```python
from build123d import *

# Parameters (mm, degrees)
BOSS_EXTRUDE1_DEPTH = 200
SKETCH2_R           = 2.5
CUT_EXTRUDE2_DEPTH  = 15
CUT_EXTRUDE3_START  = -15
SKETCH3_R           = 2.5
CUT_EXTRUDE3_DEPTH  = 15


with BuildPart() as part:
    # Sketch1 → Boss-Extrude1 (new body)
    with BuildSketch(Plane.XY):
        Polygon((-119, 208), (-131, 208), (-131, 42.5), (-119, 42.5), (-119, 165), align=None)
    extrude(amount=BOSS_EXTRUDE1_DEPTH)

    # Sketch2 → Cut-Extrude2 (cut)
    with BuildSketch(Plane(origin=(0, 208, 0), x_dir=(1, 0, 0), z_dir=(0, 1, 0))):
        with Locations(Location((-125, -25, 0), (0, 0, 270))):
            Circle(SKETCH2_R)
        with Locations(Location((-125, -75, 0), (0, 0, 270))):
            Circle(SKETCH2_R)
        with Locations(Location((-125, -125, 0), (0, 0, 270))):
            Circle(SKETCH2_R)
        with Locations(Location((-125, -175, 0), (0, 0, 270))):
            Circle(SKETCH2_R)
    extrude(amount=-CUT_EXTRUDE2_DEPTH, mode=Mode.SUBTRACT)

    # Sketch3 → Cut-Extrude3 (cut)
    with BuildSketch(Plane.XZ.offset(-42.5).offset(CUT_EXTRUDE3_START)):
        with Locations(Location((-125, 175, 0), (0, 0, 90))):
            Circle(SKETCH3_R)
        with Locations(Location((-125, 125, 0), (0, 0, 90))):
            Circle(SKETCH3_R)
        with Locations(Location((-125, 75, 0), (0, 0, 90))):
            Circle(SKETCH3_R)
        with Locations(Location((-125, 25, 0), (0, 0, 90))):
            Circle(SKETCH3_R)
    extrude(amount=CUT_EXTRUDE3_DEPTH, mode=Mode.SUBTRACT)


solid = part.part
```
Can you work these out from the model? Positions are in its coordinate system, mm. A direction names the side the tool comes from. Coordinates: 2 decimals unless noted, no trailing zeros. Order: outer loops, then holes, each group sorted by start corner. A loop starts at its lowest first (then second) coordinate and runs counter-clockwise, first axis right, second up. Notation, with made-up numbers: (74.25, -38) -> (106.25, -38) arc R13 ccw to (106.25, -13) -> close; hole circle Ø5 at (-4, -10.5). An arc over 180 degrees is marked (long way). Write each question's results on one line, items separated by ' | '.
Item 1: If I drill on line 1 along Z through (x, y) = (-125, 48); line 2 along X through (y, z) = (200, 175); line 3 along Z through (x, y) = (-123.25, 52.5), over which ranges is the centre line in solid material (lowest first)?
Results are:
line 1: 0 to 22.5, 27.5 to 72.5, 77.5 to 122.5, 127.5 to 172.5, 177.5 to 200 | line 2: -131 to -127.5, -122.5 to -119 | line 3: 0 to 23.21, 26.79 to 73.21, 76.79 to 123.21, 126.79 to 173.21, 176.79 to 200
Item 2: If we mould it in two halves opening along X, with no side actions, what happens to faces 1 (the face through (-125, 193, 25)), 2 (the face through (-125, 193, 75)), 3 (the face through (-131, 126, 99)), 4 (the face through (-125, 208, 99))? For each: +X half, -X half, draft (parallel to the pull), parting line (faces both ways), or undercut.
Results are:
face 1: undercut | face 2: undercut | face 3: -X half | face 4: draft
Item 3: Which directions (+Z, -Z, +X, -X, +Y, -Y) give clear straight access to the entire face, cutting with the end or side of a thin tool? Please do faces 5 (the face through (-125, 126, 200)), 6 (the face through (-125, 193, 175)), 7 (the face through (-127.48, 50.1, 74.67)).
Results are:
face 5: +Z, +X, -X, +Y, -Y | face 6: +Y | face 7: -Y
Item 4: I want a section at A-A, the plane z = 75. Write out the boundary of the cut face in (x, y), then the cut area to 3 significant figures.
Results are:
outline: (-131, 42.5) -> (-127.5, 42.5) -> (-127.5, 57.5) -> (-122.5, 57.5) -> (-122.5, 42.5) -> (-119, 42.5) -> (-119, 208) -> (-122.5, 208) -> (-122.5, 193) -> (-127.5, 193) -> (-127.5, 208) -> (-131, 208) -> close | area: 1,840 mm²
Item 5: I'm going to push flat-ended pins straight in: pin 1 Ø4 at (x, z) = (-125, 125) entering from +Y; pin 2 Ø6 at (x, z) = (-125, 125) entering from -Y; pin 3 Ø3 at (x, z) = (-125, 75) entering from -Y. Where does each tip first touch, or does it pass through?
Results are:
pin 1: y = 193 | pin 2: y = 42.5 | pin 3: y = 57.5
